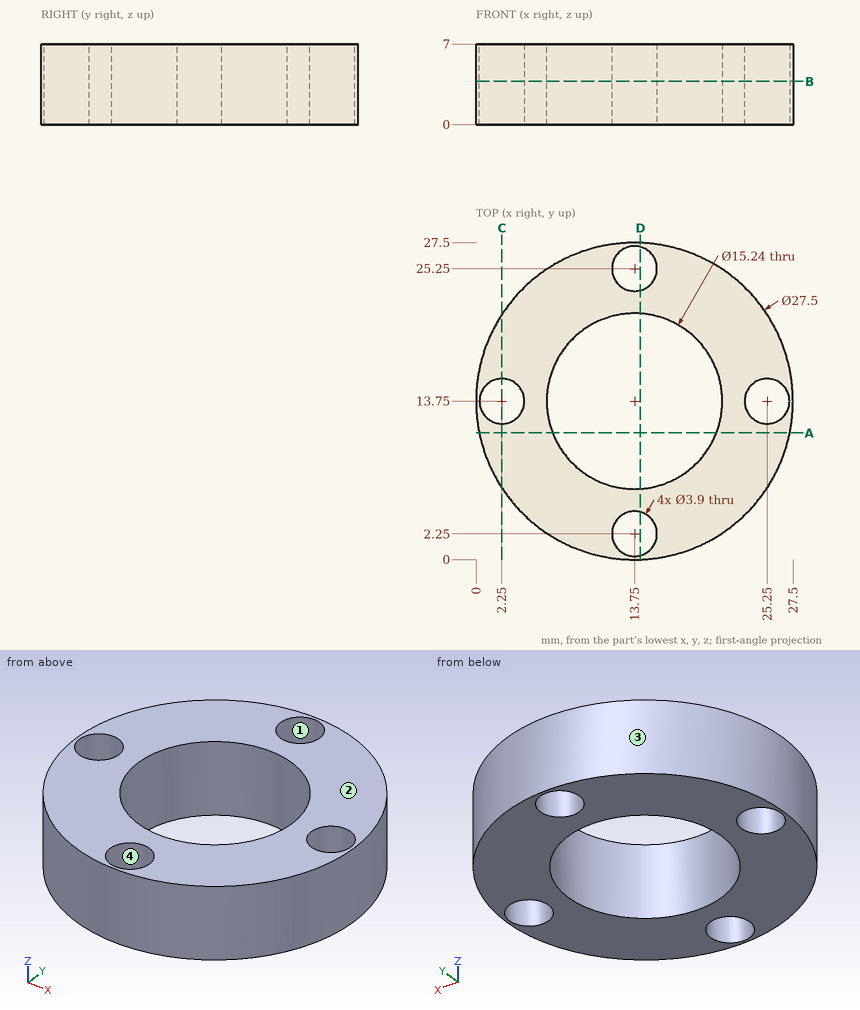
Geometry: see drawing. Coordinates: mm, zero at the bounding-box minimum. Coordinates: 2 decimals unless noted, no trailing zeros. Order: outer loops, then holes, each group sorted by start corner. A loop starts at its lowest first (then second) coordinate and runs counter-clockwise, first axis right, second up. Notation, with made-up numbers: M 61,-23 L 80,-23 A18 cw 80,6 Z; hole C 8,59.25 d5. An arc over 180 degrees is marked long. Answer in a Markdown table with one row per item. Add a question column.
Q1. Mould query, pull axis Y, two halves, no side actions, for the marked faces 1, 2, 3 and 4. Classes: released by +Y, released by -Y, zero draft, split by the parting line, or undercut.
Q2. Section query D-D on x = 14.25. Return the cut outline in (y, z), and give its area (3 significant figures).
Q3. Section query A-A on y = 11. Return the cut outline in (x, z).
Q4. Section query B-B on z = 3.75. Return the cut outline in (x, y).
Q5. Line query: L1, parallel to Y at x = 13.75, z = 4.5; L2, parallel to X at y = 24.25, z = 2; L3, parallel to Y at x = 10.5, z = 4.75. Output: solid intervals per line, ascending.
Q6. Section query C-C on x = 2.25. Return the cut outline in (y, z), and give its area (3 significant figures).
Q7. Contact query for flat-ended pins moving along their axis: P1, Ø1.5, axis at x = 12, z = 1, coming from the -Y side; P2, Ø3, axis at x = 25.25, y = 13.75, coming from the -Z side; P3, Ø3, axis at x = 5.5, z = 6, coming from the -Y side; P4, Ø3, axis at y = 3, z = 6, coming from the +X side. Output: stop coordinate, or through.
Completed:
| question | item | result |
|---|---|---|
| 1 | face 1 | undercut |
| 1 | face 2 | zero draft |
| 1 | face 3 | split by the parting line |
| 1 | face 4 | undercut |
| 2 | outline | M 0.01,0 L 0.37,0 L 0.37,7 L 0.01,7 Z; M 4.13,0 L 6.15,0 L 6.15,7 L 4.13,7 Z; M 21.35,0 L 23.37,0 L 23.37,7 L 21.35,7 Z; M 27.13,0 L 27.49,0 L 27.49,7 L 27.13,7 Z |
| 2 | area | 33.1 mm2 |
| 3 | outline | M 0.28,0 L 6.64,0 L 6.64,7 L 0.28,7 Z; M 20.86,0 L 27.22,0 L 27.22,7 L 20.86,7 Z |
| 4 | outline | C 13.75,13.75 d27.5; hole C 2.25,13.75 d3.9; hole C 13.75,13.75 d15.24; hole C 13.75,2.25 d3.9; hole C 13.75,25.25 d3.9; hole C 25.25,13.75 d3.9 |
| 5 | L1 | y = 0 to 0.3, 4.2 to 6.13, 21.37 to 23.3, 27.2 to 27.5 |
| 5 | L2 | x = 4.87 to 12.08, 15.42 to 22.63 |
| 5 | L3 | y = 0.39 to 6.86, 20.64 to 27.11 |
| 6 | outline | M 6.21,0 L 11.8,0 L 11.8,7 L 6.21,7 Z; M 15.7,0 L 21.29,0 L 21.29,7 L 15.7,7 Z |
| 6 | area | 78.2 mm2 |
| 7 | P1 | stops at y = 0.04 |
| 7 | P2 | passes through |
| 7 | P3 | stops at y = 1.77 |
| 7 | P4 | stops at x = 23.92 |
